Autodesk Inventor part; units mm, degrees
ref_plane "YZ Plane" through (0, 0, 0) normal (1, 0, 0) x (0, 1, 0)
ref_plane "XZ Plane" through (0, 0, 0) normal (0, 1, 0) x (-1, 0, 0)
ref_plane "XY Plane" through (0, 0, 0) normal (0, 0, 1) x (1, 0, 0)
sketch "Sketch1" plane through (0, 0, 0) normal (0, 1, 0) x (-1, 0, 0)
  circle A0 centre (0, 0) radius 1.55
  circle A1 centre (0, 0) radius 4.5
  dimension "d0" = 3.1
  dimension "d1" = 9
extrude "Extrusion1" add sketch "Sketch1" along normal blind 12
sketch "Sketch2" plane through (0, 0, 0) normal (0, 1, 0) x (-1, 0, 0)
  line L0 (4.825, 0) -> (-4.825, 0)
  line L1 (-4.825, 0) -> (-4.825, 10)
  line L2 (-4.825, 10) -> (4.825, 10)
  line L3 (4.825, 10) -> (4.825, 0)
  line L4 (2.325, 0) -> (2.325, 10)
  line L5 (-2.325, 10) -> (-2.325, 0)
  circle A0 centre (0, 0) radius 4.5
  circle A1 centre (0, 0) radius 4.5
  line L6 (2.325, 3.05) -> (-2.325, 3.05)
  circle A2 centre (0, 0) radius 1.55
  point P0 (-2.325, 3.8528)
  point P1 (2.325, 3.8528)
  point P2 (-4.5, 0)
  point P3 (4.5, 0)
  dimension "d4" = 4.65
  dimension "d5" = 2.325
  dimension "d6" = 2.5
  dimension "d7" = 2.5
  dimension "d8" = 10
  dimension "d25" = 1.5
extrude "Extrusion2" add sketch "Sketch2" along normal blind 12 contours L0 A0 L4 L2 L3 | L0 L4 A0 | A0 L5 L0 | L0 L1 L2 L5 A0
extrude "Extrusion4" cut sketch "Sketch2" along normal blind 20 contours L4 L6 L5 A0 | A2 L0 | L0 A2
sketch "Sketch3" plane through (4.825, 0, 10) normal (1, 0, 0) x (0, 0, -1)
  circle A0 centre (3.05, 3.05) radius 1.05
  circle A1 centre (3.05, 8.95) radius 1.05
  line L0 (0, 0) -> (0, 12)
  line L1 (0, 12) -> (10, 12)
  line L2 (0, 0) -> (10, 0)
  dimension "d11" = 2.1
  dimension "d12" = 2.1
  dimension "d13" = 2
  dimension "d14" = 2
  dimension "d26" = 5.9
  dimension "d27" = 3.05
extrude "Extrusion3" cut sketch "Sketch3" against normal blind 11
fillet "Fillet2" radius 2 4 edges at (4.5, 6, 0) (-4.5, 6, 0) (-4.825, 6, 0) (4.825, 6, 0)
fillet "Fillet3" radius 2 4 edges at (-3.575, 12, 10) (-3.575, 0, 10) (3.575, 0, 10) (3.575, 12, 10)
fillet "Fillet4" radius 1 16 edges at (0, 12, -4.5) (4.4886, 12, -0.6014) (-4.4886, 12, -0.6014) (-4.825, 12, 4.2892) (-4.825, 11.4142, 9.4142) (-4.825, 6, 10) (-4.825, 0.5858, 9.4142) (-4.825, 0, 4.2892) (4.4886, 0, -0.6014) (-4.4886, 0, -0.6014) (0, 0, -4.5) (4.825, 0, 4.2892) (4.825, 0.5858, 9.4142) (4.825, 6, 10) (4.825, 11.4142, 9.4142) (4.825, 12, 4.2892)
properties part number "Feather_clip_acrylic"
Part model, mm, in its own coordinate system. A direction names the side the tool comes from. Round coordinates to 2 decimals unless told otherwise and drop trailing zeros. Write each loop counter-clockwise with the first axis right and the second up, starting at its lowest first coordinate (ties: lowest second). Pieces come first, ordered by that corner, then holes. Notation, with made-up numbers: M 35,-3 L 62,-3 A23 ccw 62,8 Z; hole C 54.25,25.5 d1. An arc over 180 degrees is marked long. One line per question, with ' | ' between items.
(1) Saw through at A-A on y = 3.05. Write the cut outline in (x, z) (3 decimals).
Answer key:
outline: M -4.825,0.578 A2 ccw -4.601,-0.342 A2 cw -4.414,-0.874 A4.5 ccw 4.414,-0.874 A2 cw 4.601,-0.342 A2 ccw 4.825,0.578 L 4.825,5.9 L 2.325,5.9 L 2.325,3.05 L -2.325,3.05 L -2.325,5.9 L -4.825,5.9 Z; M -4.825,8 L -2.325,8 L -2.325,10 L -3.825,10 A1 ccw -4.825,9 Z; M 2.325,8 L 4.825,8 L 4.825,9 A1 ccw 3.825,10 L 2.325,10 Z; hole C 0,0 d3.1
(2) 3-axis set-ups, long thin cutter, end or side, ignore diameter. For faces 5 (the face through (0, 12, 2)), 6 (the face through (2.325, 6, 7)): which of +Z, -Z, +X, -X, +Y, -Y reach the whole face in a straight line?
Answer key:
face 5: +Z, -Z, +X, -X, +Y | face 6: +Z, +Y, -Y
(3) Pin check, flat tips, straight feed: pin 1 (3.5 mm diameter, centred on x = 0.5, y = 7, fed in from +Z); pin 2 (4 mm diameter, centred on x = 2.5, y = 8.5, fed in from -Z). Stop position of each tip, or through.
Answer key:
pin 1: stops at z = 3.05 | pin 2: stops at z = -4.47
(4) Saw through at C-C on z = 6.95. Write the cut outline in (x, y) (3 decimals).
Answer key:
outline: M -4.825,1 A1 ccw -3.825,0 L -2.325,0 L -2.325,2 L -4.825,2 Z; M -4.825,4.1 L -2.325,4.1 L -2.325,7.9 L -4.825,7.9 Z; M -4.825,10 L -2.325,10 L -2.325,12 L -3.825,12 A1 ccw -4.825,11 Z; M 2.325,0 L 3.825,0 A1 ccw 4.825,1 L 4.825,2 L 2.325,2 Z; M 2.325,4.1 L 4.825,4.1 L 4.825,7.9 L 2.325,7.9 Z; M 2.325,10 L 4.825,10 L 4.825,11 A1 ccw 3.825,12 L 2.325,12 Z
(5) Saw through at B-B on x = 0. Write the cut outline in (y, z).
Answer key:
outline: M 0,-3.5 A1 ccw 1,-4.5 L 11,-4.5 A1 ccw 12,-3.5 L 12,-1.55 L 0,-1.55 Z; M 0,1.55 L 12,1.55 L 12,3.05 L 0,3.05 Z
(6) Probe line 1 along Y through (x, z) = (2.95, 6.95); line 2 along X through (y, z) = (5, 5.5) (3 decimals); line 3 along X through (y, z) = (7.75, -0.25). List the from-to ranges inside material, lowest first.
Answer key:
line 1: y = 0 to 2, 4.1 to 7.9, 10 to 12 | line 2: x = -4.825 to -2.325, 2.325 to 4.825 | line 3: x = -4.65 to -1.53, 1.53 to 4.65
(7) Two-plate mould, pull along Y, no slides. Class faces 1 (the face through (3.59, 8.31, 7.78)), 2 (the face through (4.524, 11.715, 4.237)), 3 (the face through (-3.56, 8.31, 7.78)), 4 (the face through (0, 6, 3.05)): released by +Y, released by -Y, zero draft, split by the parting line, or undercut.
Answer key:
face 1: undercut | face 2: released by +Y | face 3: undercut | face 4: zero draft
